Work out the finished part from the listing and answer in its coordinate system (mm). A direction names the side the tool comes from. Give positions to 0.01 mm unless a question says otherwise; leave off trailing zeros. Order: outer loops, then holes, each group sorted by start corner. A loop starts at its lowest first (then second) coordinate and runs counter-clockwise, first axis right, second up. Notation, with made-up numbers: (56, -8) -> (93, -8) arc R23 ccw to (93, 11) -> close; hole circle Ø7 at (68.25, 7). An arc over 180 degrees is marked (long way). Answer as CSV lines item,"result". Start each with the question number.
1. A cutting plane is placed at A-A (x = 23.5). Give the vertices of the cut face in (y, z), then the cut area to 3 significant figures.
2. For faces 1 (the flat face through (8, 6, 1)), 2 (the flat face through (-23.1, 3.9, 0.5)), 3 (the cylindrical face through (-0.485, -31.564, 0.493)), 4 (the flat face through (18.18, 63.98, 0.49)), determine the directions among +Z, -Z, +X, -X, +Y, -Y from which every point of the face is accessible in a straight line to the end or side of a thin tool.
3. For a pull along Y with two mould halves and no side action, classify faces 5 (the flat face through (-23.128, -9.285, 0.493)), 6 (the flat face through (8, 6, 0)), 7 (the flat face through (-3.4, 63.66, 0.49)) as released by +Y, released by -Y, zero draft, split by the parting line, or undercut.
4. A flat-ended cylindrical pin translates along its axis: pin 1 (0.5 mm diameter, centred on y = 10, z = 0.5, fed in from -X). Find the tip coordinate at first contact, or state that the pin passes through.
5. A cutting plane is placed at D-D (x = -25). Give the vertices of the cut face in (y, z).
6. Find the intervals of material crossed by L1, parallel to X at y = 13.5, z = 0.1; L2, parallel to X at y = -18.5, z = 0.4; L3, parallel to Y at x = -16, z = 0.2, in increasing order.
7. A cutting plane is placed at C-C (y = 56.5). Give the vertices of the cut face in (x, z).
8. A cutting plane is placed at B-B (z = 0.7). Give the vertices of the cut face in (x, y).
from build123d import *

# Parameters (mm, degrees)
F1_DEPTH = 1


# Not quite as in the source:
# - ends of sketch curves that miss each other by under 0.0002 mm in the source are joined


with BuildPart() as f1:
    # F0 (on Top) → F1 (new body)
    with BuildSketch(Plane.XY):
        Polygon((28.8763996214, 52.6419393718), (20.6990148872, 75), (15.5881475657, 52.6419393718), (0, 52.6419393718), (-6.8996730261, 75), (-14.0548860654, 52.6419393718), (-32.458178699, 52.6419393718), (-32.458178699, 17.8880356252), (-14.0548860654, 7.6663014479), (-32.458178699, 0), (-14.0548860654, -5.889575201), (-32.458178699, -12.7771692351), (-32.458178699, -38.8200990856), (50, -38.8200990856), (50, 52.6419393718), align=None)
        with BuildLine():
            ThreePointArc((-6.6301580518, 24.9263830483), (-0.2351544327, 31.911792251), (6.0177850537, 24.7989334166))
            Line((6.0177850537, 24.7989334166), (6.0177850537, -24.9158367515))
            ThreePointArc((6.0177850537, -24.9158367515), (-0.631557079, -31.5651788842), (-7.2808992118, -24.9158367515))
            Line((-7.2808992118, -24.9158367515), (-6.6301580518, 24.9263830483))
        make_face(mode=Mode.SUBTRACT)
        with BuildLine():
            ThreePointArc((20.0069602579, 23.4479047358), (26.4433873817, 29.1369264448), (32.8798145056, 23.4479047358))
            Line((32.8798145056, 23.4479047358), (32.8798145056, -25.096591562))
            ThreePointArc((32.8798145056, -25.096591562), (26.443391107, -31.5330224112), (20.0069602579, -25.096591562))
            Line((20.0069602579, -25.096591562), (20.0069602579, 23.4479047358))
        make_face(mode=Mode.SUBTRACT)
    extrude(amount=F1_DEPTH)


solid = f1.part
Answer sheet:
1,outline,"(-38.82, 0) -> (-30.82, 0) -> (-30.82, 1) -> (-38.82, 1) -> close; (28.43, 0) -> (67.34, 0) -> (67.34, 1) -> (28.43, 1) -> close"
1,area,"46.9 mm^2"
2,face 1,"+Z, +X, -X, +Y, -Y"
2,face 2,"+Z, -Z, -X"
2,face 3,"+Z, -Z"
2,face 4,"+Z, -Z, +Y"
3,face 5,"undercut"
3,face 6,"zero draft"
3,face 7,"released by +Y"
4,pin 1,"stops at x = -18.71"
5,outline,"(-38.82, 0) -> (-9.99, 0) -> (-9.99, 1) -> (-38.82, 1) -> close; (-2.39, 0) -> (3.11, 0) -> (3.11, 1) -> (-2.39, 1) -> close; (13.75, 0) -> (52.64, 0) -> (52.64, 1) -> (13.75, 1) -> close"
6,L1,"x = -24.56 to -6.78, 6.02 to 20.01, 32.88 to 50"
6,L2,"x = -32.46 to -7.2, 6.02 to 20.01, 32.88 to 50"
6,L3,"y = -38.82 to -6.62, -5.27 to 6.86, 8.75 to 52.64"
7,outline,"(-12.82, 0) -> (-1.19, 0) -> (-1.19, 1) -> (-12.82, 1) -> close; (16.47, 0) -> (27.47, 0) -> (27.47, 1) -> (16.47, 1) -> close"
8,outline,"(-32.46, -38.82) -> (50, -38.82) -> (50, 52.64) -> (28.88, 52.64) -> (20.7, 75) -> (15.59, 52.64) -> (0, 52.64) -> (-6.9, 75) -> (-14.05, 52.64) -> (-32.46, 52.64) -> (-32.46, 17.89) -> (-14.05, 7.67) -> (-32.46, 0) -> (-14.05, -5.89) -> (-32.46, -12.78) -> close; hole (-7.28, -24.92) arc R6.65 ccw to (6.02, -24.92) -> (6.02, 24.8) arc R6.36 ccw (long way) to (-6.63, 24.93) -> close; hole (20.01, -25.1) arc R6.44 ccw to (32.88, -25.1) -> (32.88, 23.45) arc R6.49 ccw to (20.01, 23.45) -> close"
